Part model, mm, in its own coordinate system. A direction names the side the tool comes from. Round coordinates to 2 decimals unless told otherwise and drop trailing zeros. Write each loop counter-clockwise with the first axis right and the second up, starting at its lowest first coordinate (ties: lowest second). Pieces come first, ordered by that corner, then holes. Notation, with made-up numbers: M 56,63.25 L 103,63.25 A16 cw 103,67.25 Z; hole C 89,85 d9. An arc over 180 degrees is marked long. Answer as a JSON object with one key per item and string values. Group by question number.
1. Two-plate mould, pull along Z, no slides. Class faces 4 (the face through (52, -42.5, -170)), 5 (the face through (92.4, -32.4, -156.9)), 6 (the face through (5, 1, -87)), 7 (the face through (4, 1, -168)): +Z half, -Z half, draft (parallel to the pull), parting line (faces both ways), or undercut.
2. Which spindle directions (+Z, -Z, +X, -X, +Y, -Y) get a long thin tool onto all of the face, cutting with end or side? Do faces 1 (the face through (25.754, 0.187, -2.465)), 2 (the face through (87, 22.5, -72)), 3 (the face through (85, 1, -85)). Say none if no direction does.
3. Band-saw the part on A-A, the plane z = -144.5. Write the cut outline in (x, y).
4. Band-saw the part on C-C, the plane x = 30. Count the separate pieces of the cut face and the enclosed holes in it, plus the area to 4 significant figures.
5. Drill centre lines: line 1 (Y direction, x = 75, z = -1.95); line 2 (X direction, y = 11, z = -109); line 3 (Z direction, x = 72, y = -9). Where is each one in solid material? Low to high. Write a range as from..to.
6. Band-saw the part on B-B, the plane y = -8. Write the cut outline in (x, z).
7. Drop flat-ended pins along their axis: pin 1 (5 mm diameter, centred on x = 85.5, y = 33.5, fed in from -Z); pin 2 (2 mm diameter, centred on y = 20, z = -64.5, fed in from +X); pin 3 (2 mm diameter, centred on x = 92, z = -97, fed in from +Y). Give the stop position or say it passes through.
from build123d import *

# Parameters (mm, degrees)
SKETCH1_W           = 65
SKETCH1_H           = 162
BOSS_EXTRUDE1_DEPTH = 42.5
CUT_EXTRUDE1_DEPTH  = 206.949629764
SKETCH4_R           = 4.25
CUT_EXTRUDE2_DEPTH  = 5
SKETCH5_W           = 2
SKETCH5_H           = 65
CUT_EXTRUDE3_DEPTH  = 206.949629919


with BuildPart() as part:
    # Sketch1 → Boss-Extrude1 (new, symmetric)
    with BuildSketch(Plane(origin=(0, 0, 0), x_dir=(1, 0, 0), z_dir=(0, 1, 0))):
        Polygon((100, 5), (100, 167), (105, 172), (0, 172), (5, 167), (5, 5), (0, 5), (0, 0), (105, 0), (105, 5), align=None)
        with Locations((52.5, 86)):
            Rectangle(SKETCH1_W, SKETCH1_H, mode=Mode.SUBTRACT)
    extrude(amount=BOSS_EXTRUDE1_DEPTH, both=True)

    # Sketch2 → Cut-Extrude1 (cut, through all)
    with BuildSketch(Plane(origin=(0, 0, 0), x_dir=(0, 0, -1), z_dir=(1, 0, 0))):
        Polygon((0, 22.5), (147, 22.5), (167, 42.5), (0, 42.5), align=None)
    cut_extrude1 = extrude(amount=CUT_EXTRUDE1_DEPTH, mode=Mode.SUBTRACT)

    # Mirror1: Cut-Extrude1 across plane
    add(cut_extrude1.mirror(Plane.ZX), mode=Mode.SUBTRACT)

    # Sketch3 → section 0 of cut_loft1
    with BuildSketch(Plane(origin=(0, 0, -170), x_dir=(-1, 0, 0), z_dir=(0, 0, -1)), mode=Mode.PRIVATE) as cut_loft1_s0:
        with BuildLine():
            Line((-102.5, 40), (0, 40))
            Line((0, 40), (0, -40))
            Line((0, -40), (-102.5, -40))
            Line((-102.5, -40), (-102.5, 40))
        make_face()
    # loft up to a face of the part (cut_loft1)
    loft([cut_loft1_s0.sketch, part.faces().sort_by_distance((52.5, 0, -172))[0]], mode=Mode.SUBTRACT)

    # Sketch4 → Cut-Extrude2 (cut)
    with BuildSketch(Plane.XY):
        with Locations((30, 0)):
            Circle(SKETCH4_R)
        with Locations((75, 0)):
            Circle(SKETCH4_R)
    extrude(amount=-CUT_EXTRUDE2_DEPTH, mode=Mode.SUBTRACT)

    # Sketch5 → Cut-Extrude3 (cut, through all)
    with BuildSketch(Plane(origin=(0, 0, 0), x_dir=(0, 0, -1), z_dir=(1, 0, 0))):
        with Locations((171, 0)):
            Rectangle(SKETCH5_W, SKETCH5_H)
    extrude(amount=CUT_EXTRUDE3_DEPTH, mode=Mode.SUBTRACT)


solid = part.part
Worked answers:
{
 "1": {"face 4": "draft", "face 5": "+Z half", "face 6": "undercut", "face 7": "undercut"},
 "2": {"face 1": "+Z", "face 2": "+Z, +X, -X, +Y", "face 3": "+Y, -Y"},
 "3": {"outline": "M 5,-22.5 L 20,-22.5 L 20,22.5 L 5,22.5 Z; M 85,-22.5 L 100,-22.5 L 100,22.5 L 85,22.5 Z"},
 "4": {"separate pieces": "3", "enclosed holes": "0", "area": "442.5 mm^2"},
 "5": {"line 1": "y = -22.5..-4.25, 4.25..22.5", "line 2": "x = 5..20, 85..100", "line 3": "z = -170..-167, -5..0"},
 "6": {"outline": "M 0,-5 L 5,-5 L 5,-167 L 2,-170 L 103,-170 L 100,-167 L 100,-5 L 105,-5 L 105,0 L 0,0 Z; hole M 20,-167 L 85,-167 L 85,-5 L 20,-5 Z"},
 "7": {"pin 1": "stops at z = -170", "pin 2": "stops at x = 100", "pin 3": "stops at y = 22.5"}
}
